Here's how the part is built. I have some questions about the finished solid (model axes, mm). Face numbers are marked on the shaded views. A direction names the side the tool comes from. Round coordinates to 2 decimals unless told otherwise and drop trailing zeros. Write each loop counter-clockwise with the first axis right and the second up, starting at its lowest first coordinate (ties: lowest second). Pieces come first, ordered by that corner, then holes. Notation, with made-up numbers: M 40,78.5 L 52,78.5 A30 cw 52,100.5 Z; hole C 34.25,-11 d3. An arc over 180 degrees is marked long. Write item = value, one per line. Start each with the question number.
(1) I want a section at B-B (x = 18.5). List the corners of the cut face in (y, z) for me, and give its area (3 significant figures).
(2) I want a section at C-C (x = 34.5). List the corners of the cut face in (y, z) for me.
(3) I want a section at A-A (z = -50). List the corners of the cut face in (x, y) for me.
(4) On a 3-axis mill with a long thin cutter (end or side, diameter ignored), from which of +Z, -Z, +X, -X, +Y, -Y can I reach the whole of each face in a straight line? I mean the marked faces 5, 6 and 7. Say none if no direction works.
(5) I want a section at D-D (z = -34). List the corners of the cut face in (x, y) for me.
(6) I need wall thicknesses on line 1 along X through (y, z) = (2.4, -20); line 2 along Z through (x, y) = (19, 1.9); line 3 along X through (y, z) = (2.6, -47.5). Which ranges of each line are inside material? Lowest first, please.
(7) Will these pins go through, and if not, where does the flat tip stop? pin 1 Ø1.5 at (y, z) = (4, -32) entering from -X; pin 2 Ø1.5 at (y, z) = (4.5, -19) entering from +X; pin 3 Ø1.5 at (y, z) = (2, -24) entering from +X.
(8) If we mould it in two halves opening along Z, with no side actions, what happens to the marked faces 1, 2, 3 and 4? For each: released by +Z, released by -Z, zero draft, split by the parting line, or undercut.
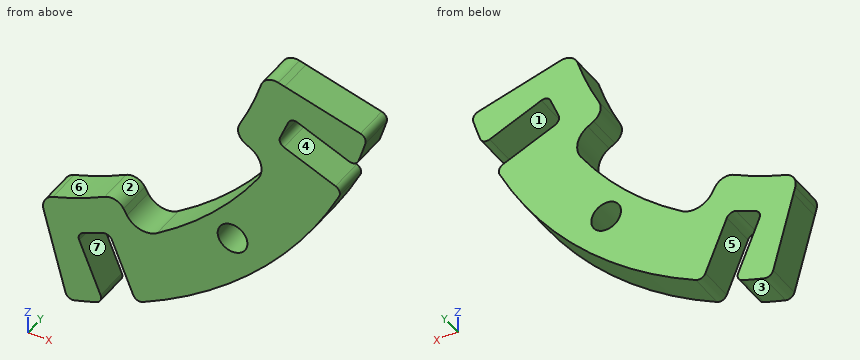
```python
from build123d import *

# Parameters (mm, degrees)
SKETCH1_R                       = 60
SKETCH1_R_2                     = 45
BOSS_EXTRUDE1_DEPTH             = 5
CUT_EXTRUDE1_DEPTH              = 6
CIRPATTERN1_COUNT               = 8
SKETCH3_R                       = 2.1
CUT_EXTRUDE2_DEPTH              = 6
CIRPATTERN2_COUNT               = 4
SKIZZE1_OUTSIDE_W               = 155.956
SKIZZE1_OUTSIDE_H               = 155.956
SCHNITT_LINEAR_AUSTRAGEN1_DEPTH = 6
VERRUNDUNG1_R                   = 1
SCHNITT_LINEAR_AUSTRAGEN2_DEPTH = 6
VERRUNDUNG2_R                   = 1
KREISMUSTER1_COUNT              = 2
KREISMUSTER1_ANGLE              = 45
VERRUNDUNG2_OF_KREISMUSTER1_R   = 1


with BuildPart() as part:
    # Sketch1 → Boss-Extrude1 (new body)
    with BuildSketch(Plane(origin=(0, 0, 0), x_dir=(1, 0, 0), z_dir=(0, 1, 0))):
        Circle(SKETCH1_R)
        Circle(SKETCH1_R_2, mode=Mode.SUBTRACT)
    extrude(amount=BOSS_EXTRUDE1_DEPTH)

    # Sketch2 → Cut-Extrude1 (cut, through all)
    with BuildSketch(Plane(origin=(0, 5, 0), x_dir=(1, 0, 0), z_dir=(0, 1, 0))):
        with BuildLine():
            Line((12.399026137, 46.273795509), (12.153476553, 45.357391985))
            ThreePointArc((12.153476553, 45.357391985), (12.332388249, 43.876840862), (13.485952537, 42.931679261))
            Line((13.485952537, 42.931679261), (-13.485952537, 42.931679261))
            ThreePointArc((-13.485952537, 42.931679261), (-12.332388249, 43.876840862), (-12.153476553, 45.357391985))
            Line((-12.153476553, 45.357391985), (-12.399026137, 46.273795509))
            ThreePointArc((-12.399026137, 46.273795509), (-12.051156799, 48.63074892), (-10.0950767, 49.990893435))
            ThreePointArc((-10.0950767, 49.990893435), (0, 51), (10.0950767, 49.990893435))
            ThreePointArc((10.0950767, 49.990893435), (12.051156799, 48.63074892), (12.399026137, 46.273795509))
        make_face()
    cut_extrude1 = extrude(amount=-CUT_EXTRUDE1_DEPTH, mode=Mode.SUBTRACT)

    # CirPattern1: Cut-Extrude1 ×8 about axis
    cirpattern1_axis = Axis((0, 0, 0), (0, 1, 0))
    for i in range(1, CIRPATTERN1_COUNT):
        add(cut_extrude1.rotate(cirpattern1_axis, i * 360 / CIRPATTERN1_COUNT), mode=Mode.SUBTRACT)

    # Sketch3 → Cut-Extrude2 (cut, through all)
    with BuildSketch(Plane(origin=(0, 5, 0), x_dir=(1, 0, 0), z_dir=(0, 1, 0))):
        with Locations((38.890872965, 38.890872965)):
            Circle(SKETCH3_R)
    cut_extrude2 = extrude(amount=-CUT_EXTRUDE2_DEPTH, mode=Mode.SUBTRACT)

    # CirPattern2: Cut-Extrude2 ×4 about axis
    cirpattern2_axis = Axis((0, 0, 0), (0, 1, 0))
    for i in range(1, CIRPATTERN2_COUNT):
        add(cut_extrude2.rotate(cirpattern2_axis, i * 360 / CIRPATTERN2_COUNT), mode=Mode.SUBTRACT)

    # Skizze1 outside → Schnitt-Linear austragen1 (cut, through all)
    with BuildSketch(Plane(origin=(0, 5, 0), x_dir=(1, 0, 0), z_dir=(0, 1, 0))):
        Rectangle(SKIZZE1_OUTSIDE_W, SKIZZE1_OUTSIDE_H)
        Polygon((0, 0), (24.798052275, 92.547591019), (92.547591019, 24.798052275), align=None, mode=Mode.SUBTRACT)
    extrude(amount=-SCHNITT_LINEAR_AUSTRAGEN1_DEPTH, mode=Mode.SUBTRACT)

    # Verrundung1
    verrundung1_edges = [part.edges().sort_by_distance(p)[0] for p in [
        (57.955549577, 2.5, -15.529142706),
        (15.529142706, 2.5, -57.955549577),
    ]]
    fillet(verrundung1_edges, radius=VERRUNDUNG1_R)

    # Skizze2 → Schnitt-Linear austragen2 (cut, through all)
    with BuildSketch(Plane(origin=(0, 5, 0), x_dir=(1, 0, 0), z_dir=(0, 1, 0))):
        Polygon((16.824472787, 47.150685206), (21.44387045, 45.237268045), (25.270704773, 54.47606337), (20.651307111, 56.389480532), align=None)
    schnitt_linear_austragen2 = extrude(amount=-SCHNITT_LINEAR_AUSTRAGEN2_DEPTH, mode=Mode.SUBTRACT)

    # Verrundung2
    verrundung2_edges = [part.edges().sort_by_distance(p)[0] for p in [
        (20.631367024, 2.5, -56.341340903),
        (25.250764686, 2.5, -54.427923741),
        (16.824472787, 2.5, -47.150685206),
        (21.44387045, 2.5, -45.237268045),
    ]]
    fillet(verrundung2_edges, radius=VERRUNDUNG2_R)

    # Kreismuster1: Schnitt-Linear austragen2 ×2 about axis
    kreismuster1_axis = Axis((0, 0, 0), (0, -1, 0))
    for i in range(1, KREISMUSTER1_COUNT):
        add(schnitt_linear_austragen2.rotate(kreismuster1_axis, i * KREISMUSTER1_ANGLE / (KREISMUSTER1_COUNT - 1)), mode=Mode.SUBTRACT)

    # Verrundung2 of Kreismuster1
    verrundung2_of_kreismuster1_edges = [part.edges().sort_by_distance(p)[0] for p in [
        (54.427923741, 2.5, -25.250764686),
        (56.341340903, 2.5, -20.631367024),
        (45.237268045, 2.5, -21.44387045),
        (47.150685206, 2.5, -16.824472787),
    ]]
    fillet(verrundung2_of_kreismuster1_edges, radius=VERRUNDUNG2_OF_KREISMUSTER1_R)


solid = part.part
```
Returned:
q1.outline = M 0,-57.08 L 5,-57.08 L 5,-51.2 L 0,-51.2 Z; M 0,-46.46 L 5,-46.46 L 5,-41.02 L 0,-41.02 Z
q1.area = 56.6 mm²
q2.outline = M 0,-49.09 L 5,-49.09 L 5,-37.56 L 0,-37.56 Z
q3.outline = M 13.4,0 L 18,0 L 18,5 L 13.4,5 Z; M 23.42,0 L 33.17,0 L 33.17,5 L 23.42,5 Z
q4.face_5 = -Z, +Y, -Y
q4.face_6 = +Z, -X, +Y, -Y
q4.face_7 = +Y, -Y
q5.outline = M 38.01,0 L 49.44,0 L 49.44,5 L 38.01,5 Z
q6.line_1 = 40.31 to 45.84, 54.82 to 56.47
q6.line_2 = -56.91 to -52.4, -46.25 to -40.79
q6.line_3 = 12.73 to 17.15, 22.38 to 36.66
q7.pin_1 = 39.1
q7.pin_2 = 57.16
q7.pin_3 = 53.22
q8.face_1 = undercut
q8.face_2 = released by +Z
q8.face_3 = released by -Z
q8.face_4 = undercut
